```python
from build123d import *

# Parameters (mm, degrees)
SKETCH_13_W         = 21.5
SKETCH_13_H         = 3
CUT_EXTRUDE_9_DEPTH = 2.5
CHAMFER_1_SIZE      = 1.75


with BuildPart() as part:
    # Sketch 1 → Revolve 1 (revolve)
    with BuildSketch(Plane.XY, mode=Mode.PRIVATE) as revolve_1_sk:
        Polygon((0, 92.035042223), (0, 67.035042223), (6, 67.035042223), (6, 86.035042223), (10.75, 90.785042223), (10.75, 92.035042223), align=None)
    revolve(revolve_1_sk.sketch.rotate(Axis((0, 125.763182898, 0), (0, -1, 0)), 180), axis=Axis((0, 125.763182898, 0), (0, -1, 0)))

    # Sketch 13 → Cut-Extrude 9 (cut)
    with BuildSketch(Plane(origin=(0, 92.035042223, 0), x_dir=(-1, 0, 0), z_dir=(0, 1, 0))):
        Rectangle(SKETCH_13_W, SKETCH_13_H)
    extrude(amount=-CUT_EXTRUDE_9_DEPTH, mode=Mode.SUBTRACT)

    # Chamfer 1
    chamfer_1_edges = [part.edges().sort_by_distance(p)[0] for p in [
        (6, 67.035042223, 0),
    ]]
    chamfer(chamfer_1_edges, length=CHAMFER_1_SIZE)


solid = part.part
```
CAD build for the part. Positions are in the model's coordinates, mm. A direction names the side the tool comes from. Coordinates: 2 decimals unless noted, no trailing zeros. Order: outer loops, then holes, each group sorted by start corner. A loop starts at its lowest first (then second) coordinate and runs counter-clockwise, first axis right, second up.
(1) Saw through at B-B, the plane z = 0. Write the cut outline in (x, y), and give its area (3 significant figures).
Solution:
outline: (-9.5, 89.54) - (-6, 86.04) - (-6, 68.79) - (-4.25, 67.04) - (4.25, 67.04) - (6, 68.79) - (6, 86.04) - (9.5, 89.54) - close
area: 279 mm2
(2) Mould opens along Z. For faces 1 (the face through (0, 89.535, 0)), 2 (the face through (0.215, 91.419, 10.748)), 3 (the face through (-5.723, 77.531, -1.802)) say: released by +Z, released by -Z, zero draft, split by the parting line, or undercut.
Solution:
face 1: undercut
face 2: released by +Z
face 3: split by the parting line
(3) Saw through at C-C, the plane y = 78.75. Write the cut outline in (x, z), and give its area (3 significant figures).
Solution:
outline: circle Ø12 at (0, 0)
area: 113 mm2
(4) Pin check, flat tips, straight feed: pin 1 Ø2 at (y, z) = (84.5, -1.5) entering from +X; pin 2 Ø1.5 at (x, z) = (-3, -0.5) entering from +Y; pin 3 Ø6 at (y, z) = (73, -2.5) entering from -X. Stop position of each tip, or through.
Solution:
pin 1: stops at x = 5.98
pin 2: stops at y = 89.54
pin 3: stops at x = -6
(5) Drill centre lines: L1, parallel to Z at x = 0, y = 89.75; L2, parallel to Y at x = -1, z = -0.5; L3, parallel to Z at x = 1.5, y = 77.5. Where is each one in solid material? Low to high.
Solution:
L1: z = -9.71 to -1.5, 1.5 to 9.71
L2: y = 67.04 to 89.54
L3: z = -5.81 to 5.81
(6) Which spindle directions (+Z, -Z, +X, -X, +Y, -Y) get a long thin tool onto all of the face, cutting with end or side? Do faces 4 (the face through (0, 91, -1.5)), 5 (the face through (0, 67.035, 0)). Say none if no direction does.
Solution:
face 4: +X, -X, +Y
face 5: +Z, -Z, +X, -X, -Y
(7) Saw through at A-A, the plane x = 0. Write the cut outline in (y, z).
Solution:
outline: (67.04, -4.25) - (68.79, -6) - (86.04, -6) - (90.79, -10.75) - (92.04, -10.75) - (92.04, -1.5) - (89.54, -1.5) - (89.54, 1.5) - (92.04, 1.5) - (92.04, 10.75) - (90.79, 10.75) - (86.04, 6) - (68.79, 6) - (67.04, 4.25) - close
